Source: CAD feature listing. Evaluate the final solid. Frame: model axes, mm. A direction names the side the tool comes from. Give positions to 0.01 mm unless a question says otherwise; leave off trailing zeros. Order: outer loops, then holes, each group sorted by start corner. A loop starts at its lowest first (then second) coordinate and runs counter-clockwise, first axis right, second up.
from build123d import *

# Parameters (mm, degrees)
SKETCH1_W           = 26
SKETCH1_H           = 40
SKETCH1_R           = 4.4
BOSS_EXTRUDE1_DEPTH = 2
SKETCH2_W           = 11.5
SKETCH2_H           = 17
SKETCH2_R           = 4.4
BOSS_EXTRUDE2_DEPTH = 2
SKETCH3_W           = 26
SKETCH3_H           = 40
SKETCH3_W_2         = 23
SKETCH3_H_2         = 37
BOSS_EXTRUDE3_DEPTH = 8
SKETCH4_R           = 2
CUT_EXTRUDE1_DEPTH  = 2


with BuildPart() as part:
    # Sketch1 → Boss-Extrude1 (new body)
    with BuildSketch(Plane.XY):
        with Locations((13, -20)):
            Rectangle(SKETCH1_W, SKETCH1_H)
        with Locations((13, -26.5)):
            Circle(SKETCH1_R, mode=Mode.SUBTRACT)
    extrude(amount=BOSS_EXTRUDE1_DEPTH)

    # Sketch2 → Boss-Extrude2 (add)
    with BuildSketch(Plane.XY.offset(2)):
        with Locations((13, -26.5)):
            Rectangle(SKETCH2_W, SKETCH2_H)
        with Locations((13, -26.5)):
            Circle(SKETCH2_R, mode=Mode.SUBTRACT)
    extrude(amount=BOSS_EXTRUDE2_DEPTH)

    # Sketch3 → Boss-Extrude3 (add)
    with BuildSketch(Plane.XY.offset(2)):
        with Locations((13, -20)):
            Rectangle(SKETCH3_W, SKETCH3_H)
        with Locations((13, -20)):
            Rectangle(SKETCH3_W_2, SKETCH3_H_2, mode=Mode.SUBTRACT)
    extrude(amount=BOSS_EXTRUDE3_DEPTH)

    # Sketch4 → Cut-Extrude1 (cut)
    with BuildSketch(Plane.XZ.offset(40)):
        with Locations(Location((13, 5, 0), (0, 0, 270))):
            Circle(SKETCH4_R)
    extrude(amount=-CUT_EXTRUDE1_DEPTH, mode=Mode.SUBTRACT)


solid = part.part
(1) Section D-D, the plane z = 5. Return loops of the section in (x, y).
(2) Section C-C, the plane y = -2.5. Return loops of the section in (x, z).
(3) Line query: line 1 along Y through (x, z) = (13, 2.6); line 2 along X through (y, z) = (-36, 4); line 3 along Y through (x, z) = (18.75, 7.25). Output: solid intervals per line, ascending.
(4) Section B-B, the plane x = 13. Return loops of the section in (y, z), plus the area to 3 significant figures.
(5) Draft query along X for faces 3 (the flat face through (26, -20, 5)), 4 (the cylindrical face through (15, -39, 5)), 5 (the flat face through (13, 0, 5)). Return one class per face: +X half, -X half, draft (parallel to the pull), parting line (faces both ways), or undercut.
(6) Access query for faces 1 (the flat face through (18.75, -27, 3)), 2 (the flat face through (1, -20, 10)). Directions: +Z, -Z, +X, -X, +Y, -Y. A direction counts if a zero-diameter tool reaches every point of the face in a straight line with its end or side. Return the directions, or none.
(7) Pin query (flat end, axial travel): pin 1 Ø1.5 at (x, y) = (4.5, -25) entering from +Z; pin 2 Ø6 at (x, y) = (10.5, -22.5) entering from +Z. Return the tip coordinate at first contact, or that it passes through.
(8) Section A-A, the plane y = -26.5. Return loops of the section in (x, z).
Checks:
1. outline: (0, -40) - (11, -40) - (11, -38.5) - (1.5, -38.5) - (1.5, -1.5) - (24.5, -1.5) - (24.5, -38.5) - (15, -38.5) - (15, -40) - (26, -40) - (26, 0) - (0, 0) - close
2. outline: (0, 0) - (26, 0) - (26, 10) - (24.5, 10) - (24.5, 2) - (1.5, 2) - (1.5, 10) - (0, 10) - close
3. line 1: y = -40 to -38.5, -35 to -30.9, -22.1 to -18, -1.5 to 0
3. line 2: x = 0 to 1.5, 24.5 to 26
3. line 3: y = -40 to -38.5, -1.5 to 0
4. outline: (-40, 0) - (-30.9, 0) - (-30.9, 4) - (-35, 4) - (-35, 2) - (-38.5, 2) - (-38.5, 3) - (-40, 3) - close; (-40, 7) - (-38.5, 7) - (-38.5, 10) - (-40, 10) - close; (-22.1, 0) - (0, 0) - (0, 10) - (-1.5, 10) - (-1.5, 2) - (-18, 2) - (-18, 4) - (-22.1, 4) - close
4. area: 96.8 mm2
5. face 3: +X half
5. face 4: undercut
5. face 5: draft
6. face 1: +Z
6. face 2: +Z, +X, -X, +Y, -Y
7. pin 1: stops at z = 2
7. pin 2: stops at z = 4
8. outline: (0, 0) - (8.6, 0) - (8.6, 4) - (7.25, 4) - (7.25, 2) - (1.5, 2) - (1.5, 10) - (0, 10) - close; (17.4, 0) - (26, 0) - (26, 10) - (24.5, 10) - (24.5, 2) - (18.75, 2) - (18.75, 4) - (17.4, 4) - close
